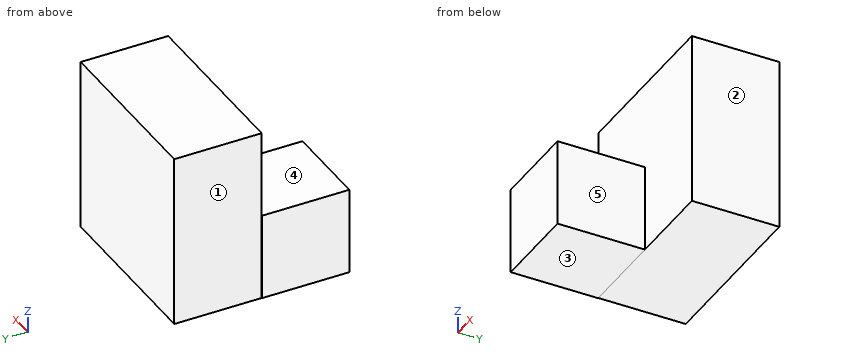
from build123d import *

# Parameters (mm, degrees)
F1_W     = 50.79394
F1_H     = 50.793938
F2_DEPTH = 25.4
F0_W     = 25.396969
F0_H     = 25.396969
F3_DEPTH = 25.4


with BuildPart() as f2:
    # F1 (on Front) → F2 (new body)
    with BuildSketch(Plane.XZ):
        with Locations((-50.884868, -50.602984)):
            Rectangle(F1_W, F1_H)
    extrude(amount=-F2_DEPTH)

    # F0 (on Front) → F3 (join)
    with BuildSketch(Plane.XZ):
        with Locations((-63.683377, -63.301468)):
            Rectangle(F0_W, F0_H)
    extrude(amount=F3_DEPTH)


solid = f2.part
Geometry: final body of the model. Coordinates: model frame, mm. Face numbers are marked on the shaded views. A direction names the side the tool comes from. Coordinates: 2 decimals unless noted, no trailing zeros. Order: outer loops, then holes, each group sorted by start corner. A loop starts at its lowest first (then second) coordinate and runs counter-clockwise, first axis right, second up. Notation, with made-up numbers: (38, 79) - (44, 79) arc R26 cw to (44, 113) - close; hole circle Ø2 at (76, 5.25). An arc over 180 degrees is marked (long way). Use one line per item in the form item = value.
1) Section C-C (y = -15). Return loops of the section in (x, z), then the cut area to 3 significant figures.
Solutions:
outline = (-76.38, -76) - (-50.98, -76) - (-50.98, -50.6) - (-76.38, -50.6) - close
area = 645 mm^2
2) Section B-B (z = -66). Return loops of the section in (x, y), then the cut area to 3 significant figures.
Solutions:
outline = (-76.38, -25.4) - (-50.98, -25.4) - (-50.98, 0) - (-25.49, 0) - (-25.49, 25.4) - (-76.28, 25.4) - (-76.28, 0) - (-76.38, 0) - close
area = 1,940 mm^2
3) Set-up query: the marked faces 1, 2, 3, 4 and 5. Return all of +Z, -Z, +X, -X, +Y, -Y with unobstructed straight access to the full face (end or side cutting, diameter ignored); none if empty.
Solutions:
face_1 = +Z, -Z, -X, +Y
face_2 = +Z, -Z, +X, +Y, -Y
face_3 = -Z, +X, -X, +Y, -Y
face_4 = +Z, +X, -X, -Y
face_5 = +Z, -Z, +X, -Y
4) Pin query (flat end, axial travel): pin 1 (10 mm diameter, centred on x = -65, z = -37.5, fed in from -Y); pin 2 (1.5 mm diameter, centred on y = -15, z = -57.5, fed in from +X); pin 3 (20.5 mm diameter, centred on x = -62, y = -15, fed in from +Z). Return the tip coordinate at first contact, or that it passes through.
Solutions:
pin_1 = 0
pin_2 = -50.98
pin_3 = -50.6
5) Section A-A (x = -60). Return loops of the section in (y, z), then the cut area to 3 significant figures.
Solutions:
outline = (-25.4, -76) - (25.4, -76) - (25.4, -25.21) - (0, -25.21) - (0, -50.6) - (-25.4, -50.6) - close
area = 1,940 mm^2
6) Ray query, L1, parallel to X at y = 6.5, z = -66; L2, parallel to X at y = -4.5, z = -51.5; L3, parallel to Y at x = -54, z = -35. Return the intervals inside material, ascending.
Solutions:
L1 = -76.28 to -25.49
L2 = -76.38 to -50.98
L3 = 0 to 25.4
7) Section D-D (x = -46). Return loops of the section in (y, z).
Solutions:
outline = (0, -76) - (25.4, -76) - (25.4, -25.21) - (0, -25.21) - close
